Could you check a few things on this model? Use its own coordinates, in mm. Round coordinates to 2 decimals unless told otherwise and drop trailing zeros. Loops run counter-clockwise (first coordinate to the right, second up) from the corner with the lowest first, then second, coordinate; pieces in that order, holes last.
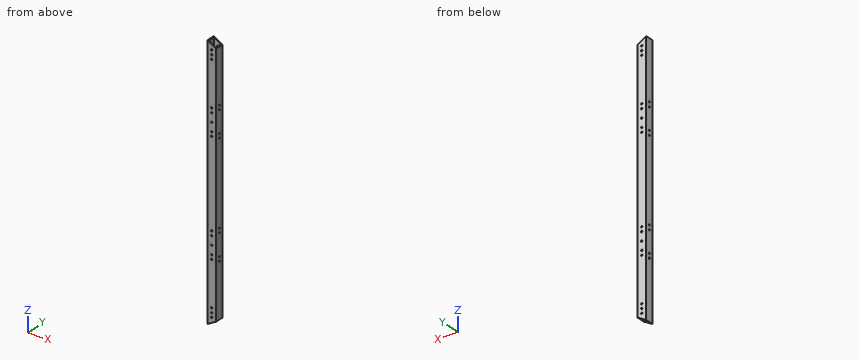
from build123d import *

# Parameters (mm, degrees)
SKETCH_1_W          = 20
SKETCH_1_H          = 20
SKETCH_1_W_2        = 16
SKETCH_1_H_2        = 16
EXTRUDE_1_DEPTH     = 600
CUT_EXTRUDE_1_DEPTH = 300
SKETCH_3_R          = 1.65
CUT_EXTRUDE_2_DEPTH = 300
SKETCH_4_R          = 1.65
CUT_EXTRUDE_3_DEPTH = 10
SKETCH_6_R          = 1.65
CUT_EXTRUDE_4_DEPTH = 601.416522091


with BuildPart() as part:
    # 草图1 → 凸台-拉伸1 (new body)
    with BuildSketch(Plane.XY):
        Rectangle(SKETCH_1_W, SKETCH_1_H)
        Rectangle(SKETCH_1_W_2, SKETCH_1_H_2, mode=Mode.SUBTRACT)
    extrude(amount=EXTRUDE_1_DEPTH)

    # 草图2 → 切除-拉伸1 (cut, symmetric)
    with BuildSketch(Plane(origin=(0, 10, 0), x_dir=(1, 0, 0), z_dir=(0, 1, 0))):
        Polygon((-10, 0), (10, -11.547005384), (10, 0), align=None)
        Polygon((10, -600), (-10, -600), (10, -588.452994616), align=None)
    extrude(amount=CUT_EXTRUDE_1_DEPTH, both=True, mode=Mode.SUBTRACT)

    # 草图3 → 切除-拉伸2 (cut, symmetric)
    with BuildSketch(Plane(origin=(0, 10, 0), x_dir=(1, 0, 0), z_dir=(0, 1, 0))):
        with Locations(Location((0, -17.318286674, 0), (0, 0, 270))):
            Circle(SKETCH_3_R)
        with Locations(Location((0, -582.681713326, 0), (0, 0, 270))):
            Circle(SKETCH_3_R)
        with Locations(Location((0, -27.318286674, 0), (0, 0, 270))):
            Circle(SKETCH_3_R)
        with Locations(Location((0, -37.318286674, 0), (0, 0, 270))):
            Circle(SKETCH_3_R)
        with Locations(Location((0, -562.681713326, 0), (0, 0, 270))):
            Circle(SKETCH_3_R)
        with Locations(Location((0, -572.681713326, 0), (0, 0, 270))):
            Circle(SKETCH_3_R)
    extrude(amount=CUT_EXTRUDE_2_DEPTH, both=True, mode=Mode.SUBTRACT)

    # 草图4 → 切除-拉伸3 (cut, symmetric)
    with BuildSketch(Plane(origin=(0, 0, 0), x_dir=(1, 0, 0), z_dir=(0, 1, 0))):
        with Locations(Location((0, -169.998286674, 0), (0, 0, 270))):
            Circle(SKETCH_4_R)
        with Locations(Location((0, -429.998286674, 0), (0, 0, 270))):
            Circle(SKETCH_4_R)
        with Locations(Location((0, -149.998286674, 0), (0, 0, 270))):
            Circle(SKETCH_4_R)
        with Locations(Location((0, -189.998286674, 0), (0, 0, 270))):
            Circle(SKETCH_4_R)
        with Locations(Location((0, -409.998286674, 0), (0, 0, 270))):
            Circle(SKETCH_4_R)
        with Locations(Location((0, -449.998286674, 0), (0, 0, 270))):
            Circle(SKETCH_4_R)
        with Locations(Location((0, -199.998286674, 0), (0, 0, 270))):
            Circle(SKETCH_4_R)
        with Locations(Location((0, -139.998286674, 0), (0, 0, 270))):
            Circle(SKETCH_4_R)
        with Locations(Location((0, -459.998286674, 0), (0, 0, 270))):
            Circle(SKETCH_4_R)
        with Locations(Location((0, -399.998286674, 0), (0, 0, 270))):
            Circle(SKETCH_4_R)
    extrude(amount=CUT_EXTRUDE_3_DEPTH, both=True, mode=Mode.SUBTRACT)

    # 草图6 → 切除-拉伸4 (cut, through all)
    with BuildSketch(Plane.ZY.offset(10)):
        with Locations((195, 0)):
            Circle(SKETCH_6_R)
        with Locations((145, 0)):
            Circle(SKETCH_6_R)
        with Locations((205, 0)):
            Circle(SKETCH_6_R)
        with Locations((135, 0)):
            Circle(SKETCH_6_R)
        with Locations((465, 0)):
            Circle(SKETCH_6_R)
        with Locations((395, 0)):
            Circle(SKETCH_6_R)
        with Locations((455, 0)):
            Circle(SKETCH_6_R)
        with Locations((405, 0)):
            Circle(SKETCH_6_R)
    extrude(amount=-CUT_EXTRUDE_4_DEPTH, mode=Mode.SUBTRACT)


solid = part.part
Item 1: Will these pins go through, and if not, where does the flat tip stop? pin 1 (5 mm diameter, centred on x = 6, y = 0, fed in from -Z); pin 2 (4 mm diameter, centred on x = 0, z = 430, fed in from +Y).
Results list:
pin 1: stops at z = 10.39
pin 2: stops at y = 10
Item 2: If I drill on line 1 along Y through (x, z) = (7.5, 411); line 2 along Y through (x, z) = (9, 145), over which ranges is the centre line in solid material (lowest first)?
Results list:
line 1: y = -10 to -8, 8 to 10
line 2: y = -10 to -1.65, 1.65 to 10
Item 3: If we section it at B-B, the plane x = -4.75: Please give me the cut outline in (y, z).
Results list:
outline: (-10, 3.03) - (-8, 3.03) - (-8, 596.97) - (-10, 596.97) - close; (8, 3.03) - (10, 3.03) - (10, 596.97) - (8, 596.97) - close
Item 4: If we section it at A-A, the plane z = 553: Please give me the cut outline in (x, y), then the cut area to 3 significant figures.
Results list:
outline: (-10, -10) - (10, -10) - (10, 10) - (-10, 10) - close; hole (-8, -8) - (8, -8) - (8, 8) - (-8, 8) - close
area: 144 mm2
